```python
from build123d import *

# Parameters (mm, degrees)
F0_R     = 6.35
F1_DEPTH = 76.2
F2_T     = -2.54
F5_R     = 6.35
F5_R_2   = 5.3717360651
F6_DEPTH = 25.4


# Not quite as in the source:
# - the program builds the solid bodies; features that only make, move or delete a surface that nothing else refers to are left out


with BuildPart() as f1:
    # F0 (on Top) → F1 (new body)
    with BuildSketch(Plane.XY):
        Circle(F0_R)
    extrude(amount=F1_DEPTH)

    # F2
    f2_openings = [f1.faces().sort_by_distance(p)[0] for p in [
        (0, 0, 76.2),
    ]]
    offset(amount=F2_T, openings=f2_openings)

    # F5 (on face) → F6 (cut)
    with BuildSketch(Plane.XY.offset(76.2)):
        Circle(F5_R)
        Circle(F5_R_2, mode=Mode.SUBTRACT)
    extrude(amount=-F6_DEPTH, mode=Mode.SUBTRACT)


solid = f1.part
```
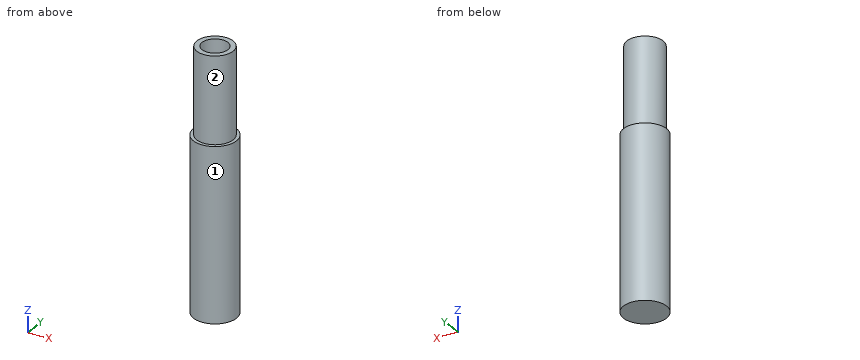
Check sheet for the modelled part. Datum: model origin and axes. Units: mm. Face numbers are marked on the shaded views. A direction names the side the tool comes from. Coordinates: 2 decimals unless noted, no trailing zeros. Loops run counter-clockwise (first coordinate to the right, second up) from the corner with the lowest first, then second, coordinate; pieces in that order, holes last. Notation, with made-up numbers: M 77,-39 L 111,-39 A14 cw 111,-21 Z; hole C 0,12.25 d4. An arc over 180 degrees is marked long. Answer as a JSON object with one key per item and string values.
1. Depth check by flat-ended pin: P1, Ø1.5, axis at y = 4, z = 49.5, coming from the +X side; P2, Ø2, axis at y = 4.5, z = 14, coming from the -X side; P3, Ø1, axis at y = 2, z = 27, coming from the +X side. Enter the tip coordinate at first touch or a pass-through.
Outcome:
{"P1": "x = 5.46", "P2": "x = -5.3", "P3": "x = 6.17"}
2. Sectioned sample at A-A on x = 0. Record the cut outline in (y, z).
Outcome:
{"outline": "M -6.35,0 L 6.35,0 L 6.35,50.8 L 5.37,50.8 L 5.37,76.2 L 3.81,76.2 L 3.81,2.54 L -3.81,2.54 L -3.81,76.2 L -5.37,76.2 L -5.37,50.8 L -6.35,50.8 Z"}
3. Scan lines: L1, parallel to Y at x = 0, z = 60.5; L2, parallel to Y at x = 0, z = 44; L3, parallel to X at y = -1.5, z = 46. Record each from-to range of solid material in increasing order. Write a range as from..to.
Outcome:
{"L1": "-5.37..-3.81, 3.81..5.37", "L2": "-6.35..-3.81, 3.81..6.35", "L3": "-6.17..-3.5, 3.5..6.17"}
4. Access from +Z, -Z, +X, -X, +Y, -Y to the whole of each face (thin tool, end or side, straight path). Record for the marked faces 1 and 2.
Outcome:
{"face 1": "+Z, -Z", "face 2": "+Z"}
5. Sectioned sample at C-C on z = 13.5. Record the cut outline in (x, y), and give its area (3 significant figures).
Outcome:
{"outline": "C 0,0 d12.7; hole C 0,0 d7.62", "area": "81.1 mm²"}
